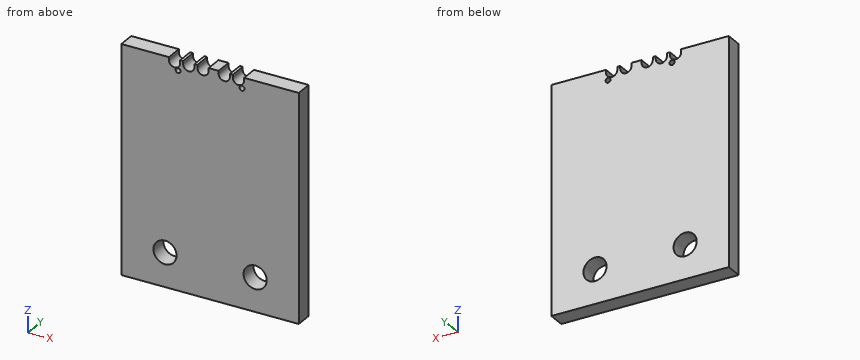
```python
from build123d import *

# Parameters (mm, degrees)
SKETCH1_R           = 0.7
SKETCH1_R_2         = 3.2639
BOSS_EXTRUDE1_DEPTH = 4.7625


with BuildPart() as part:
    # Sketch1 → Boss-Extrude1 (new body)
    with BuildSketch(Plane(origin=(0, 0, 0), x_dir=(1, 0, 0), z_dir=(0, 1, 0))):
        with BuildLine():
            Line((16, 1.185131266), (16, 65))
            Line((16, 65), (66, 65))
            Line((66, 65), (66, 1.185131266))
            Line((66, 1.185131266), (50.5875, 1.185131266))
            Line((50.5875, 1.185131266), (50.5875, 2.009827459))
            ThreePointArc((50.5875, 2.009827459), (49, 3.597327459), (47.4125, 2.009827459))
            Line((47.4125, 2.009827459), (47.4125, 1.185131266))
            Line((47.4125, 1.185131266), (46.5875, 1.185131266))
            Line((46.5875, 1.185131266), (46.5875, 2.009827459))
            ThreePointArc((46.5875, 2.009827459), (45, 3.597327459), (43.4125, 2.009827459))
            Line((43.4125, 2.009827459), (43.4125, 1.185131266))
            Line((43.4125, 1.185131266), (40.5875, 1.185131266))
            Line((40.5875, 1.185131266), (40.5875, 2.009827459))
            ThreePointArc((40.5875, 2.009827459), (39, 3.597327459), (37.4125, 2.009827459))
            Line((37.4125, 2.009827459), (37.4125, 1.185131266))
            Line((37.4125, 1.185131266), (36.5875, 1.185131266))
            Line((36.5875, 1.185131266), (36.5875, 2.009827459))
            ThreePointArc((36.5875, 2.009827459), (35, 3.597327459), (33.4125, 2.009827459))
            Line((33.4125, 2.009827459), (33.4125, 1.185131266))
            Line((33.4125, 1.185131266), (32.5875, 1.185131266))
            Line((32.5875, 1.185131266), (32.5875, 2.009827459))
            ThreePointArc((32.5875, 2.009827459), (31, 3.597327459), (29.4125, 2.009827459))
            Line((29.4125, 2.009827459), (29.4125, 1.185131266))
            Line((29.4125, 1.185131266), (16, 1.185131266))
        make_face()
        with Locations((32, 4.197327459)):
            Circle(SKETCH1_R, mode=Mode.SUBTRACT)
        with Locations((53.7, 55.426122104)):
            Circle(SKETCH1_R_2, mode=Mode.SUBTRACT)
        with Locations((28.3, 55.426122104)):
            Circle(SKETCH1_R_2, mode=Mode.SUBTRACT)
        with Locations((50, 4.197327459)):
            Circle(SKETCH1_R, mode=Mode.SUBTRACT)
    extrude(amount=-BOSS_EXTRUDE1_DEPTH)


solid = part.part
```
Part model, mm, in its own coordinate system. Give positions to 0.01 mm unless a question says otherwise; leave off trailing zeros. Loops run counter-clockwise (first coordinate to the right, second up) from the corner with the lowest first, then second, coordinate; pieces in that order, holes last. Notation, with made-up numbers: M 89,46.25 L 131,46.25 A38 ccw 131,85.25 Z; hole C 42,-9 d6. An arc over 180 degrees is marked long. Return JSON: item names as keys, results as strings.
1) Drill centre lines: line 1 (X direction, y = -3.85, z = -4); line 2 (Z direction, x = 28.3, y = -3.75); line 3 (Z direction, x = 32, y = -1.9). Where is each one in solid material? Low to high.
Calculated:
{"line 1": "x = 16 to 31.33, 32.67 to 49.33, 50.67 to 66", "line 2": "z = -65 to -58.69, -52.16 to -1.19", "line 3": "z = -65 to -4.9, -3.5 to -3.24"}
2) Saw through at B-B, the plane y = -2.7. List the corners of the cut face in (x, z) (1 decimal), then the cut area to 3 significant figures.
Calculated:
{"outline": "M 16,-65 L 66,-65 L 66,-1.2 L 50.6,-1.2 L 50.6,-2 A1.6 cw 47.4,-2 L 47.4,-1.2 L 46.6,-1.2 L 46.6,-2 A1.6 cw 43.4,-2 L 43.4,-1.2 L 40.6,-1.2 L 40.6,-2 A1.6 cw 37.4,-2 L 37.4,-1.2 L 36.6,-1.2 L 36.6,-2 A1.6 cw 33.4,-2 L 33.4,-1.2 L 32.6,-1.2 L 32.6,-2 A1.6 cw 29.4,-2 L 29.4,-1.2 L 16,-1.2 Z; hole C 28.3,-55.4 d6.5; hole C 32,-4.2 d1.4; hole C 50,-4.2 d1.4; hole C 53.7,-55.4 d6.5", "area": "3,090 mm2"}
3) Saw through at A-A, the plane x = 28.3. List the corners of the cut face in (y, z).
Calculated:
{"outline": "M -4.76,-65 L 0,-65 L 0,-58.69 L -4.76,-58.69 Z; M -4.76,-52.16 L 0,-52.16 L 0,-1.19 L -4.76,-1.19 Z"}
4) Saw through at C-C, the plane x = 54. List the corners of the cut face in (y, z).
Calculated:
{"outline": "M -4.76,-65 L 0,-65 L 0,-58.68 L -4.76,-58.68 Z; M -4.76,-52.18 L 0,-52.18 L 0,-1.19 L -4.76,-1.19 Z"}
5) Saw through at D-D, the plane x = 45. List the corners of the cut face in (y, z), then the cut area to 3 significant figures.
Calculated:
{"outline": "M -4.76,-65 L 0,-65 L 0,-3.6 L -4.76,-3.6 Z", "area": "292 mm2"}
